from build123d import *

# Parameters (mm, degrees)
IZIM1_W                     = 300
IZIM1_H                     = 50
Y_KSEKLIK_EKSTR_ZYON1_DEPTH = 10
IZIM2_R                     = 1.55
IZIM2_W                     = 120
IZIM2_H                     = 10
KES_EKSTR_ZYON1_DEPTH       = 10


with BuildPart() as part:
    # Çizim1 → Yükseklik-Ekstrüzyon1 (new body)
    with BuildSketch(Plane(origin=(0, 0, 0), x_dir=(1, 0, 0), z_dir=(0, 1, 0))):
        Rectangle(IZIM1_W, IZIM1_H)
    extrude(amount=Y_KSEKLIK_EKSTR_ZYON1_DEPTH)

    # Çizim2 → Kes-Ekstrüzyon1 (cut)
    with BuildSketch(Plane(origin=(0, 10, 0), x_dir=(1, 0, 0), z_dir=(0, 1, 0))):
        with Locations(Location((140, 20, 0), (0, 0, 270))):
            Circle(IZIM2_R)
        with Locations(Location((0, 20, 0), (0, 0, 270))):
            Circle(IZIM2_R)
        with Locations(Location((-140, 20, 0), (0, 0, 270))):
            Circle(IZIM2_R)
        with Locations(Location((0, -20, 0), (0, 0, 270))):
            Circle(IZIM2_R)
        with Locations(Location((-140, -20, 0), (0, 0, 270))):
            Circle(IZIM2_R)
        with Locations(Location((140, -20, 0), (0, 0, 270))):
            Circle(IZIM2_R)
        with Locations((-70, -20)):
            Rectangle(IZIM2_W, IZIM2_H)
        with Locations((70, -20)):
            Rectangle(IZIM2_W, IZIM2_H)
        with Locations((-70, 20)):
            Rectangle(IZIM2_W, IZIM2_H)
        with Locations((70, 20)):
            Rectangle(IZIM2_W, IZIM2_H)
    extrude(amount=-KES_EKSTR_ZYON1_DEPTH, mode=Mode.SUBTRACT)


solid = part.part
Geometry check sheet. Reference: the model listing, model coordinates, mm. A direction names the side the tool comes from. Give positions to 0.01 mm unless a question says otherwise; leave off trailing zeros. Loops run counter-clockwise (first coordinate to the right, second up) from the corner with the lowest first, then second, coordinate; pieces in that order, holes last.
(1) Set-up check for faces 5 (the flat face through (-71, 5, -15)), 6 (the flat face through (69, 5, 15)), 7 (the flat face through (-2, 10, 0)): record each of +Z, -Z, +X, -X, +Y, -Y from which the full face is reachable in a straight line by a thin tool's end or side.
From the geometry:
face 5: -Z, +Y, -Y
face 6: +Z, +Y, -Y
face 7: +Z, -Z, +X, -X, +Y
(2) Thickness scan on L1, parallel to X at y = 5, z = 20; L2, parallel to Z at x = 140, y = 5.5; L3, parallel to X at y = 7, z = 22. Record the ranges inside material, lowest first.
From the geometry:
L1: x = -150 to -141.55, -138.45 to -130, -10 to -1.55, 1.55 to 10, 130 to 138.45, 141.55 to 150
L2: z = -25 to -21.55, -18.45 to 18.45, 21.55 to 25
L3: x = -150 to -130, -10 to 10, 130 to 150
(3) Release check for a two-part mould opening along X. For faces 1 (the flat face through (150, 5, 0)), 2 (the flat face through (-10, 5, -20)), 3 (the flat face through (130, 5, -20)), 4 (the flat face through (-2, 0, 0)) record: released by +X, released by -X, zero draft, split by the parting line, or undercut.
From the geometry:
face 1: released by +X
face 2: undercut
face 3: undercut
face 4: zero draft
(4) Depth check by flat-ended pin: pin 1 Ø2 at (x, y) = (101, 2) entering from +Z; pin 2 Ø4 at (x, z) = (0, -20) entering from +Y; pin 3 Ø1.9 at (x, z) = (0, 20) entering from -Y; pin 4 Ø3 at (x, y) = (-88, 3) entering from -Z. Enter the tip coordinate at first touch or a pass-through.
From the geometry:
pin 1: stops at z = 15
pin 2: stops at y = 10
pin 3: passes through
pin 4: stops at z = -15
(5) Section check A-A on y = 6. Record the cut outline in (x, z).
From the geometry:
outline: (-150, -25) - (-130, -25) - (-130, -15) - (-10, -15) - (-10, -25) - (10, -25) - (10, -15) - (130, -15) - (130, -25) - (150, -25) - (150, 25) - (130, 25) - (130, 15) - (10, 15) - (10, 25) - (-10, 25) - (-10, 15) - (-130, 15) - (-130, 25) - (-150, 25) - close; hole circle Ø3.1 at (-140, -20); hole circle Ø3.1 at (-140, 20); hole circle Ø3.1 at (0, -20); hole circle Ø3.1 at (0, 20); hole circle Ø3.1 at (140, -20); hole circle Ø3.1 at (140, 20)
(6) Section check B-B on x = 55. Record the cut outline in (y, z).
From the geometry:
outline: (0, -15) - (10, -15) - (10, 15) - (0, 15) - close
